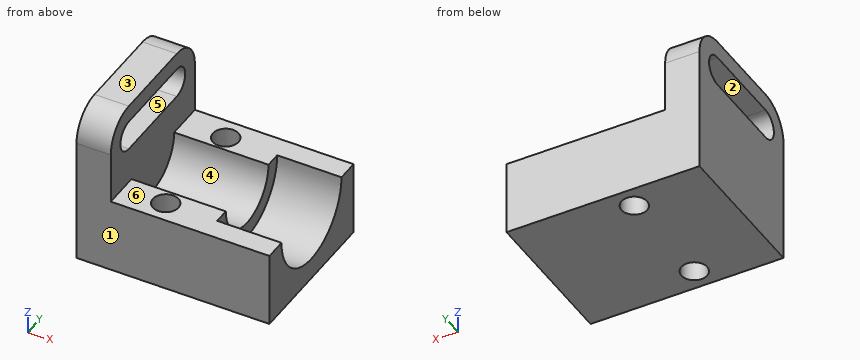
```python
from build123d import *

# Parameters (mm, degrees)
F1_DEPTH  = 35
F3_DEPTH  = 30
F5_DEPTH  = 44
F6_R      = 15
F8_DEPTH  = 16.001
F9_R      = 6
F10_DEPTH = 35.001


with BuildPart() as f1:
    # F0 (on Front) → F1 (new body, symmetric)
    with BuildSketch(Plane.XZ):
        Polygon((0, 74), (0, 0), (90, 0), (90, 35), (16, 35), (16, 74), align=None)
    extrude(amount=F1_DEPTH, both=True)

    # F2 (on face) → F3 (cut)
    with BuildSketch(Plane.YZ.offset(90)):
        with BuildLine():
            Line((25, 35), (-25, 35))
            ThreePointArc((-25, 35), (0, 10), (25, 35))
        make_face()
    extrude(amount=-F3_DEPTH, mode=Mode.SUBTRACT)

    # F4 (on face) → F5 (cut, through all)
    with BuildSketch(Plane.YZ.offset(60)):
        with BuildLine():
            Line((17.783249, 35), (-17.783249, 35))
            ThreePointArc((-17.783249, 35), (0, 17.216751), (17.783249, 35))
        make_face()
    extrude(amount=-F5_DEPTH, mode=Mode.SUBTRACT)

    # F6
    f6_edges = [f1.edges().sort_by_distance(p)[0] for p in [
        (8, -35, 74),
        (8, 35, 74),
    ]]
    fillet(f6_edges, radius=F6_R)

    # F7 (on face) → F8 (cut, through all)
    with BuildSketch(Plane.YZ.offset(16)):
        with BuildLine():
            ThreePointArc((-20, 66), (-27, 59), (-20, 52))
            Line((-20, 52), (20, 52))
            ThreePointArc((20, 52), (27, 59), (20, 66))
            Line((20, 66), (-20, 66))
        make_face()
    extrude(amount=-F8_DEPTH, mode=Mode.SUBTRACT)

    # F9 (on face) → F10 (cut, through all)
    with BuildSketch(Plane.XY.offset(35)):
        with Locations((36, -25)):
            Circle(F9_R)
        with Locations((36, 25)):
            Circle(F9_R)
    extrude(amount=-F10_DEPTH, mode=Mode.SUBTRACT)


solid = f1.part
```
The listing builds one solid part. Answer for the finished solid, in the listing's coordinates (mm). Face numbers are marked on the shaded views. A direction names the side the tool comes from. Round coordinates to 2 decimals unless told otherwise and drop trailing zeros. Write each loop counter-clockwise with the first axis right and the second up, starting at its lowest first coordinate (ties: lowest second). Pieces come first, ordered by that corner, then holes. Notation, with made-up numbers: (-25.75, 86.25) -> (-1.75, 86.25) arc R25 ccw to (-1.75, 115.25) -> close; hole circle Ø3 at (-36, -34). An arc over 180 degrees is marked (long way). Answer as a JSON object with one key per item and string values. Group by question number.
Q1. Section B-B (z = 8) is taken. Write down the section's boundary in (x, y), plus the area to 3 significant figures.
Q2. Section D-D (x = 17.5) is taken. Write down the section's boundary in (y, z), plus the area to 3 significant figures.
Q3. Section C-C (z = 53.5) is taken. Write down the section's boundary in (x, y).
Q4. Section A-A (y = 0) is taken. Write down the section's boundary in (x, z), plus the area to 3 significant figures.
Q5. Each of these flat-tipped pins is pushed along its axis until it touches: pin 1 Ø17 at (y, z) = (-15, 45) entering from +X; pin 2 Ø5 at (x, y) = (61, 30.5) entering from +Z; pin 3 Ø1 at (y, z) = (-16.5, 53.5) entering from +X; pin 4 Ø6 at (y, z) = (-20.5, 35.5) entering from +X. Where does it stop, or does it pass through?
Q6. Which of the six approach directions +Z, -Z, +X, -X, +Y, -Y give full straight-line access (tool end or side, diameter ignored) to the marked faces 4, 5 and 6?
Q7. Straight lines are drawn through the part: line 1 along Y through (x, z) = (36, 8); line 2 along Y through (x, z) = (36, 21); line 3 along Z through (x, y) = (8, -10.5). For each, find the intervals that lie inside material, in ascending order.
Q8. Determine the mould class of the marked faces 1, 2 and 3 for opening direction Z: pulls with the +Z half, pulls with the -Z half, needs draft (parallel to the pull), parting line crosses it, or undercut.
Check values:
{
 "1": {"outline": "(0, -35) -> (90, -35) -> (90, 35) -> (0, 35) -> close; hole circle Ø12 at (36, -25); hole circle Ø12 at (36, 25)", "area": "6,070 mm^2"},
 "2": {"outline": "(-35, 0) -> (35, 0) -> (35, 35) -> (17.78, 35) arc R17.78 cw to (-17.78, 35) -> (-35, 35) -> close", "area": "1,950 mm^2"},
 "3": {"outline": "(0, -35) -> (16, -35) -> (16, -24.33) -> (0, -24.33) -> close; (0, 24.33) -> (16, 24.33) -> (16, 35) -> (0, 35) -> close"},
 "4": {"outline": "(0, 0) -> (90, 0) -> (90, 10) -> (60, 10) -> (60, 17.22) -> (16, 17.22) -> (16, 52) -> (0, 52) -> close; (0, 66) -> (16, 66) -> (16, 74) -> (0, 74) -> close", "area": "2,020 mm^2"},
 "5": {"pin 1": "x = 16", "pin 2": "z = 35", "pin 3": "through", "pin 4": "x = 60"},
 "6": {"face 4": "+Z, +X", "face 5": "+X, -X", "face 6": "+Z, +X, +Y, -Y"},
 "7": {"line 1": "-35 to -31, -19 to 19, 31 to 35", "line 2": "-35 to -31, -19 to -10.97, 10.97 to 19, 31 to 35", "line 3": "0 to 52, 66 to 74"},
 "8": {"face 1": "needs draft", "face 2": "undercut", "face 3": "pulls with the +Z half"}
}
